```python
from build123d import *

# Parameters (mm, degrees)
SKETCH1_W           = 30
SKETCH1_H           = 13
BOSS_EXTRUDE1_DEPTH = 4
SKETCH2_W           = 18
SKETCH2_H           = 3
CUT_EXTRUDE1_DEPTH  = 14
SKETCH3_W           = 22
SKETCH3_H           = 13
BOSS_EXTRUDE2_DEPTH = 3
SKETCH4_R           = 1.75
CUT_EXTRUDE2_DEPTH  = 5
SKETCH7_R           = 1.75
CUT_EXTRUDE5_DEPTH  = 8


with BuildPart() as part:
    # Sketch1 → Boss-Extrude1 (new body)
    with BuildSketch(Plane(origin=(0, 0, 0), x_dir=(1, 0, 0), z_dir=(0, 1, 0))):
        with Locations((15, 6.5)):
            Rectangle(SKETCH1_W, SKETCH1_H)
    extrude(amount=BOSS_EXTRUDE1_DEPTH)

    # Sketch2 → Cut-Extrude1 (cut, through all)
    with BuildSketch(Plane.XY):
        with Locations((21, 1.5)):
            Rectangle(SKETCH2_W, SKETCH2_H)
    extrude(amount=-CUT_EXTRUDE1_DEPTH, mode=Mode.SUBTRACT)

    # Sketch3 → Boss-Extrude2 (add)
    with BuildSketch(Plane(origin=(0, 4, 0), x_dir=(1, 0, 0), z_dir=(0, 1, 0))):
        with Locations((19, 6.5)):
            Rectangle(SKETCH3_W, SKETCH3_H)
    extrude(amount=BOSS_EXTRUDE2_DEPTH)

    # Sketch4 → Cut-Extrude2 (cut, through all)
    with BuildSketch(Plane(origin=(0, 4, 0), x_dir=(1, 0, 0), z_dir=(0, 1, 0))):
        with Locations((5, 6.5)):
            Circle(SKETCH4_R)
    extrude(amount=-CUT_EXTRUDE2_DEPTH, mode=Mode.SUBTRACT)

    # Sketch7 → Cut-Extrude5 (cut, through all)
    with BuildSketch(Plane(origin=(0, 7, 0), x_dir=(1, 0, 0), z_dir=(0, 1, 0))):
        with Locations((20, 6.5)):
            Circle(SKETCH7_R)
        with Locations((26, 6.5)):
            Circle(SKETCH7_R)
    extrude(amount=-CUT_EXTRUDE5_DEPTH, mode=Mode.SUBTRACT)


solid = part.part
```
Input: part model. Units: mm. Frame: model coordinates. A direction names the side the tool comes from. Round coordinates to 2 decimals unless told otherwise and drop trailing zeros. Loops run counter-clockwise (first coordinate to the right, second up) from the corner with the lowest first, then second, coordinate; pieces in that order, holes last. Notation, with made-up numbers: (-36.75, 56.25) -> (22.25, 56.25) arc R17 ccw to (22.25, 85.25) -> close; hole circle Ø4 at (-35, -33). An arc over 180 degrees is marked (long way). Write each question's results on one line, items separated by ' | '.
1. Section A-A (x = 26). Return loops of the section in (y, z), and give its area (3 significant figures).
Geometry results:
outline: (3, -13) -> (7, -13) -> (7, -8.25) -> (3, -8.25) -> close; (3, -4.75) -> (7, -4.75) -> (7, 0) -> (3, 0) -> close | area: 38.0 mm2
2. Section D-D (z = -3). Return loops of the section in (x, y), and give its area (3 significant figures).
Geometry results:
outline: (0, 0) -> (12, 0) -> (12, 3) -> (30, 3) -> (30, 7) -> (8, 7) -> (8, 4) -> (0, 4) -> close | area: 132 mm2
3. Section C-C (y = 1.75). Return loops of the section in (x, z).
Geometry results:
outline: (0, -13) -> (12, -13) -> (12, 0) -> (0, 0) -> close; hole circle Ø3.5 at (5, -6.5)
4. Mould query, pull axis Z, two halves, no side actions, for faces 4 (the face through (15, 4, -13)), 5 (the face through (3.61, 2.03, -5.44)), 6 (the face through (0, 2, -6)). Classes: +Z half, -Z half, draft (parallel to the pull), parting line (faces both ways), or undercut.
Geometry results:
face 4: -Z half | face 5: undercut | face 6: draft
5. Section B-B (z = -6.5). Return loops of the section in (x, y), and give its area (3 significant figures).
Geometry results:
outline: (0, 0) -> (3.25, 0) -> (3.25, 4) -> (0, 4) -> close; (6.75, 0) -> (12, 0) -> (12, 3) -> (18.25, 3) -> (18.25, 7) -> (8, 7) -> (8, 4) -> (6.75, 4) -> close; (21.75, 3) -> (24.25, 3) -> (24.25, 7) -> (21.75, 7) -> close; (27.75, 3) -> (30, 3) -> (30, 7) -> (27.75, 7) -> close | area: 90.0 mm2
6. Set-up query: faces 1 (the face through (3, 4, -7)), 2 (the face through (12, 1, -6)), 3 (the face through (18.61, 5.03, -5.44)). Return all of +Z, -Z, +X, -X, +Y, -Y with unobstructed straight access to the full face (end or side cutting, diameter ignored); none if empty.
Geometry results:
face 1: +Z, -Z, -X, +Y | face 2: +Z, -Z, +X, -Y | face 3: +Y, -Y
7. First-contact query: P1, Ø4, axis at x = 20, z = -6.5, coming from the -Y side; P2, Ø5.5, axis at x = 26, z = -6.5, coming from the +Y side; P3, Ø1.5, axis at y = 1.5, z = -3.5, coming from the +X side; P4, Ø2.5, axis at x = 3.5, z = -7, coming from the +Y side. Flat tips, straight axial feed; report the tip coordinate or a pass-through.
Geometry results:
P1: y = 3 | P2: y = 7 | P3: x = 12 | P4: y = 4
8. Ray query, line 1 (X direction, y = 5.9, z = -6.5); line 2 (X direction, y = 0.95, z = -6.5); line 3 (Z direction, x = 20, y = 4.95). Return the intervals inside material, ascending. Write a range as from..to.
Geometry results:
line 1: 8..18.25, 21.75..24.25, 27.75..30 | line 2: 0..3.25, 6.75..12 | line 3: -13..-8.25, -4.75..0
